```python
from build123d import *

# Parameters (mm, degrees)
F1_DEPTH = 63.5
F2_DEPTH = 25.4
F3_DEPTH = 8.2804
F5_R     = 6.35


with BuildPart() as f1:
    # F0 (on Front) → F1 (new body, symmetric)
    with BuildSketch(Plane.XZ):
        Polygon((-41.275, -9.525), (41.275, -9.525), (41.275, 9.525), (25.780999, 9.525), (-41.275, 9.525), align=None)
    extrude(amount=F1_DEPTH, both=True)

    # F0 (on Front) → F2 (join, symmetric)
    with BuildSketch(Plane.XZ):
        with BuildLine():
            Line((25.780999, 9.525), (41.275, 9.525))
            Line((41.275, 9.525), (41.275, 28.504782))
            ThreePointArc((41.275, 28.504782), (47.109768, 40.801504), (60.325, 44.059042))
            Line((60.325, 44.059042), (60.325, 59.648656))
            add(Edge.make_bspline(
                [(56.560999, 59.868252), (57.809032, 59.80963), (59.063808, 59.736539), (60.325, 59.648656)],
                knots=[111.091867, 111.091867, 111.091867, 111.091867, 113.567541, 113.567541, 113.567541, 113.567541], degree=3))
            ThreePointArc((56.560999, 59.868252), (34.761492, 50.476785), (25.780999, 28.504782))
            Line((25.780999, 28.504782), (25.780999, 9.525))
        make_face()
        with BuildLine():
            Line((60.325, 59.648656), (60.325, 44.059042))
            Line((60.325, 44.059042), (85.725, 44.059042))
            Line((85.725, 44.059042), (85.725, 59.553043))
            Line((85.725, 59.553043), (61.62434, 59.553043))
            add(Edge.make_bspline(
                [(60.325, 59.648656), (60.757364, 59.618527), (61.190481, 59.586661), (61.62434, 59.553043)],
                knots=[113.567541, 113.567541, 113.567541, 113.567541, 114.416254, 114.416254, 114.416254, 114.416254], degree=3))
        make_face()
    extrude(amount=F2_DEPTH, both=True)

    # F0 (on Front) → F3 (join, symmetric)
    with BuildSketch(Plane.XZ):
        with BuildLine():
            add(Edge.make_bspline(
                [(-41.275, 9.525), (-41.868726, 35.994224), (0.557538, 62.498833), (56.560999, 59.868252)],
                knots=[0, 0, 0, 0, 111.091867, 111.091867, 111.091867, 111.091867], degree=3))
            Line((-41.275, 9.525), (25.780999, 9.525))
            Line((25.780999, 9.525), (25.780999, 28.504782))
            ThreePointArc((25.780999, 28.504782), (34.761492, 50.476785), (56.560999, 59.868252))
        make_face()
    extrude(amount=F3_DEPTH, both=True)

    # F0 (on Front) → F4 (revolve)
    with BuildSketch(Plane.XZ):
        Polygon((85.725, 59.553043), (85.725, 44.059042), (85.725, 38.1), (111.125, 38.1), (111.125, 66.675), (85.725, 66.675), align=None)
    revolve(axis=Axis((85.725, 0, 52.3875), (0, 0, -1)))

    # F5
    f5_edges = [f1.edges().sort_by_distance(p)[0] for p in [
        (41.275, -63.5, 0),
        (-41.275, -63.5, 0),
        (-41.275, 63.5, 0),
        (41.275, 63.5, 0),
    ]]
    fillet(f5_edges, radius=F5_R)


solid = f1.part
```
Geometry: final body of the model. Coordinates: model frame, mm. A direction names the side the tool comes from. Round coordinates to 2 decimals unless told otherwise and drop trailing zeros. Write each loop counter-clockwise with the first axis right and the second up, starting at its lowest first coordinate (ties: lowest second). Pieces come first, ordered by that corner, then holes. Notation, with made-up numbers: M -24,-24 L 27,-24 A25 ccw 27,1 Z; hole C -29.5,56 d4. An arc over 180 degrees is marked long. Answer in a Markdown table with one row per item. Add a question column.
(1) Cut plane A-A, the plane z = -2. Return the cut outline in (x, y) (3 decimals).
(2) Cut plane B-B, the plane y = 50.5. Return the cut outline in (x, z) (3 decimals).
(3) Ray query, L1, parallel to Z at x = 4, y = -26 (3 decimals); L2, parallel to Y at x = -30, z = 29.5; L3, parallel to X at y = -37.5, z = 9 (3 decimals). Return the intervals inside material, ascending.
(4) Contact query for flat-ended pins moving along their axis: pin 1 (19 mm diameter, centred on y = -20, z = 17, fed in from -X) (3 decimals); pin 2 (2 mm diameter, centred on y = 26.5, z = 32, fed in from +X); pin 3 (8 mm diameter, centred on x = 23.5, z = 53, fed in from +Y); pin 4 (5 mm diameter, centred on y = 16.5, z = 18, fed in from -X). Output: stop coordinate, or through.
(5) Reachability of faces 1 (the face through (109.95, -7.63, 52.59)), 2 (the face through (86, 0, 38.1)), 3 (the face through (25.781, 17, 19)), 4 (the face through (-3, -8.28, 30)) from +Z, -Z, +X, -X, +Y, -Y: full face, straight path, thin tool, end or side. Return the list, or none.
Established:
| question | item | result |
|---|---|---|
| 1 | outline | M -41.275,-57.15 A6.35 ccw -34.925,-63.5 L 34.925,-63.5 A6.35 ccw 41.275,-57.15 L 41.275,57.15 A6.35 ccw 34.925,63.5 L -34.925,63.5 A6.35 ccw -41.275,57.15 Z |
| 2 | outline | M -41.275,-9.525 L 41.275,-9.525 L 41.275,9.525 L -41.275,9.525 Z |
| 3 | L1 | -9.525 to 9.525 |
| 3 | L2 | -8.28 to 8.28 |
| 3 | L3 | -41.275 to 41.275 |
| 4 | pin 1 | x = -41.275 |
| 4 | pin 2 | through |
| 4 | pin 3 | y = 8.28 |
| 4 | pin 4 | x = 25.78 |
| 5 | face 1 | none |
| 5 | face 2 | -Z, +X, +Y, -Y |
| 5 | face 3 | +Z, -X, +Y |
| 5 | face 4 | +Z, -X, -Y |
